Can you work these out from the model? Positions are in its coordinate system, mm. A direction names the side the tool comes from. Round coordinates to 2 decimals unless told otherwise and drop trailing zeros. Loops run counter-clockwise (first coordinate to the right, second up) from the corner with the lowest first, then second, coordinate; pieces in that order, holes last. Notation, with made-up numbers: (36.25, -0.5) -> (74.25, -0.5) arc R27 ccw to (74.25, 35.5) -> close; hole circle Ø8 at (-35.75, 10.25). An arc over 180 degrees is marked (long way). Use a Markdown table: item, result.
from build123d import *

# Parameters (mm, degrees)
CROQUIS1_W              = 42
CROQUIS1_H              = 92.91
CROQUIS1_R              = 11.5
CROQUIS1_R_2            = 1.55
SALIENTE_EXTRUIR1_DEPTH = 4
CROQUIS2_R              = 1.55
CROQUIS2_W              = 4.2
CROQUIS2_H              = 6
CORTAR_EXTRUIR1_DEPTH   = 5
CORTAR_EXTRUIR2_DEPTH   = 5
CORTAR_EXTRUIR3_DEPTH   = 5
CORTAR_EXTRUIR4_DEPTH   = 5
CHAFL_N1_SIZE           = 4.1


with BuildPart() as part:
    # Croquis1 → Saliente-Extruir1 (new body)
    with BuildSketch(Plane(origin=(0, 0, 0), x_dir=(0, 0, -1), z_dir=(1, 0, 0))):
        with Locations((21, 46.455)):
            Rectangle(CROQUIS1_W, CROQUIS1_H)
        with Locations((21, 71.76)):
            Circle(CROQUIS1_R, mode=Mode.SUBTRACT)
        with Locations((5.5, 87.26)):
            Circle(CROQUIS1_R_2, mode=Mode.SUBTRACT)
        with Locations((36.5, 87.26)):
            Circle(CROQUIS1_R_2, mode=Mode.SUBTRACT)
        with Locations((36.5, 56.26)):
            Circle(CROQUIS1_R_2, mode=Mode.SUBTRACT)
        with Locations((5.5, 56.26)):
            Circle(CROQUIS1_R_2, mode=Mode.SUBTRACT)
    extrude(amount=SALIENTE_EXTRUIR1_DEPTH)

    # Croquis2 → Cortar-Extruir1 (cut, through all)
    with BuildSketch(Plane(origin=(4, 0, 0), x_dir=(0, 0, -1), z_dir=(1, 0, 0))):
        with Locations((3.6, 23.5)):
            Circle(CROQUIS2_R)
        with Locations((38.4, 23.5)):
            Circle(CROQUIS2_R)
        with Locations((3.6, 37)):
            Rectangle(CROQUIS2_W, CROQUIS2_H)
        with Locations((3.6, 10)):
            Rectangle(CROQUIS2_W, CROQUIS2_H)
        with Locations((38.4, 10)):
            Rectangle(CROQUIS2_W, CROQUIS2_H)
        with Locations((38.4, 37)):
            Rectangle(CROQUIS2_W, CROQUIS2_H)
    extrude(amount=-CORTAR_EXTRUIR1_DEPTH, mode=Mode.SUBTRACT)

    # Croquis3 → Cortar-Extruir2 (cut, through all)
    with BuildSketch(Plane(origin=(4, 0, 0), x_dir=(0, 0, -1), z_dir=(1, 0, 0))):
        Polygon((19.45, 0), (19.45, 2.05), (18.2, 2.05), (18.2, 4.95), (19.45, 4.95), (19.45, 7), (22.55, 7), (22.55, 4.95), (23.8, 4.95), (23.8, 2.05), (22.55, 2.05), (22.55, 0), align=None)
    extrude(amount=-CORTAR_EXTRUIR2_DEPTH, mode=Mode.SUBTRACT)

    # Croquis4 → Cortar-Extruir3 (cut, through all)
    with BuildSketch(Plane(origin=(4, 0, 0), x_dir=(0, 0, -1), z_dir=(1, 0, 0))):
        with BuildLine():
            Line((5.7, 37.878679656), (5.7, 36.121320344))
            ThreePointArc((5.7, 36.121320344), (5.710503119, 34.010608171), (3.6, 33.979099854))
            ThreePointArc((3.6, 33.979099854), (1.489496881, 34.010608171), (1.5, 36.121320344))
            Line((1.5, 36.121320344), (1.5, 37.878679656))
            ThreePointArc((1.5, 37.878679656), (1.489496881, 39.989391829), (3.6, 40.020900146))
            ThreePointArc((3.6, 40.020900146), (5.710503119, 39.989391829), (5.7, 37.878679656))
        make_face()
        with BuildLine():
            Line((40.5, 36.121320344), (40.5, 37.878679656))
            ThreePointArc((40.5, 37.878679656), (40.510503119, 39.989391829), (38.4, 40.020900146))
            ThreePointArc((38.4, 40.020900146), (36.289496881, 39.989391829), (36.3, 37.878679656))
            Line((36.3, 37.878679656), (36.3, 36.121320344))
            ThreePointArc((36.3, 36.121320344), (36.289496881, 34.010608171), (38.4, 33.979099854))
            ThreePointArc((38.4, 33.979099854), (40.510503119, 34.010608171), (40.5, 36.121320344))
        make_face()
        with BuildLine():
            Line((36.3, 9.121320344), (36.3, 10.878679656))
            ThreePointArc((36.3, 10.878679656), (36.289496881, 12.989391829), (38.4, 13.020900146))
            ThreePointArc((38.4, 13.020900146), (40.510503119, 12.989391829), (40.5, 10.878679656))
            Line((40.5, 10.878679656), (40.5, 9.121320344))
            ThreePointArc((40.5, 9.121320344), (40.510503119, 7.010608171), (38.4, 6.979099854))
            ThreePointArc((38.4, 6.979099854), (36.289496881, 7.010608171), (36.3, 9.121320344))
        make_face()
        with BuildLine():
            Line((5.7, 9.121320344), (5.7, 10.878679656))
            ThreePointArc((5.7, 10.878679656), (5.710503119, 12.989391829), (3.6, 13.020900146))
            ThreePointArc((3.6, 13.020900146), (1.489496881, 12.989391829), (1.5, 10.878679656))
            Line((1.5, 10.878679656), (1.5, 9.121320344))
            ThreePointArc((1.5, 9.121320344), (1.489496881, 7.010608171), (3.6, 6.979099854))
            ThreePointArc((3.6, 6.979099854), (5.710503119, 7.010608171), (5.7, 9.121320344))
        make_face()
    extrude(amount=-CORTAR_EXTRUIR3_DEPTH, mode=Mode.SUBTRACT)

    # Croquis5 → Cortar-Extruir4 (cut, through all)
    with BuildSketch(Plane(origin=(4, 0, 0), x_dir=(0, 0, -1), z_dir=(1, 0, 0))):
        with BuildLine():
            Line((21.678679656, 2.05), (20.321320344, 2.05))
            ThreePointArc((20.321320344, 2.05), (18.510162011, 1.811909807), (17.812069651, 3.5))
            ThreePointArc((17.812069651, 3.5), (18.028132476, 4.744252385), (19.117836757, 5.382524838))
            ThreePointArc((19.117836757, 5.382524838), (19.424850602, 6.97423962), (21, 7.35727725))
            ThreePointArc((21, 7.35727725), (22.575149398, 6.97423962), (22.882163243, 5.382524838))
            ThreePointArc((22.882163243, 5.382524838), (23.971867524, 4.744252385), (24.187930349, 3.5))
            ThreePointArc((24.187930349, 3.5), (23.489837989, 1.811909807), (21.678679656, 2.05))
        make_face()
    extrude(amount=-CORTAR_EXTRUIR4_DEPTH, mode=Mode.SUBTRACT)

    # Chaflán1
    chafl_n1_edges = [part.edges().sort_by_distance(p)[0] for p in [
        (2, 92.91, 0),
        (2, 92.91, -42),
    ]]
    chamfer(chafl_n1_edges, length=CHAFL_N1_SIZE)


solid = part.part
1. I want a section at C-C (y = 64). Please give me the cut outline in (x, z), plus the area to 3 significant figures.
Answer sheet:
| item | result |
|---|---|
| outline | (0, -42) -> (4, -42) -> (4, -29.49) -> (0, -29.49) -> close; (0, -12.51) -> (4, -12.51) -> (4, 0) -> (0, 0) -> close |
| area | 100 mm² |
2. Which directions (+Z, -Z, +X, -X, +Y, -Y) give clear straight access to the entire face, cutting with the end or side of a thin tool? Please do faces 4 (the flat face through (2, 44, 0)), 5 (the flat face through (2, 1, -19.45)), 6 (the cylindrical face through (2.03, 4.76, -23.96)).
Answer sheet:
| item | result |
|---|---|
| face 4 | +Z, +X, -X, +Y, -Y |
| face 5 | +X, -X, -Y |
| face 6 | +X, -X |
3. I need wall thicknesses on line 1 (Z direction, x = 1.8, y = 87.26); line 2 (Y direction, x = 1.95, z = -5.5); line 3 (Y direction, x = 3.65, z = -37). Which ranges of each line are inside material? Lowest first, please.
Answer sheet:
| item | result |
|---|---|
| line 1 | z = -42 to -38.05, -34.95 to -7.05, -3.95 to 0 |
| line 2 | y = 0 to 6.83, 13.17 to 33.83, 40.17 to 54.71, 57.81 to 85.71, 88.81 to 92.91 |
| line 3 | y = 0 to 6.6, 13.4 to 22.83, 24.17 to 33.6, 40.4 to 54.79, 57.73 to 85.79, 88.73 to 92.91 |
4. If we mould it in two halves opening along Z, with no side actions, what happens to faces 1 (the flat face through (2, 44, -42)), 2 (the flat face through (1.97, 90.89, -2.08)), 3 (the flat face through (2, 37, -1.5))? For each: +Z half, -Z half, draft (parallel to the pull), parting line (faces both ways), or undercut.
Answer sheet:
| item | result |
|---|---|
| face 1 | -Z half |
| face 2 | +Z half |
| face 3 | undercut |
5. Will these pins go through, and if not, where does the flat tip stop? pin 1 Ø2.5 at (y, z) = (23.5, -3.6) entering from +X; pin 2 Ø4 at (y, z) = (56.26, -5.5) entering from +X.
Answer sheet:
| item | result |
|---|---|
| pin 1 | passes through |
| pin 2 | stops at x = 4 |
6. I want a section at D-D (x = 1.2). State how many separate pieces and enclosed holes the cut face has, plus the area to 3 significant figures.
Answer sheet:
| item | result |
|---|---|
| separate pieces | 1 |
| enclosed holes | 11 |
| area | 3,270 mm² |
7. I want a section at A-A (y = 87.26). Please give me the cut outline in (x, z), plus the area to 3 significant figures.
Answer sheet:
| item | result |
|---|---|
| outline | (0, -42) -> (4, -42) -> (4, -38.05) -> (0, -38.05) -> close; (0, -34.95) -> (4, -34.95) -> (4, -7.05) -> (0, -7.05) -> close; (0, -3.95) -> (4, -3.95) -> (4, 0) -> (0, 0) -> close |
| area | 143 mm² |
8. I want a section at B-B (z = -30.5). Please give me the cut outline in (x, y).
Answer sheet:
| item | result |
|---|---|
| outline | (0, 0) -> (4, 0) -> (4, 65.28) -> (0, 65.28) -> close; (0, 78.24) -> (4, 78.24) -> (4, 92.91) -> (0, 92.91) -> close |
